from build123d import *

# Parameters (mm, degrees)
SKETCH1_W             = 60
SKETCH1_H             = 60
BOSS_EXTRUDE1_DEPTH   = 6
SKETCH2_W             = 55
SKETCH2_H             = 15.25
BOSS_EXTRUDE2_DEPTH   = 30
F_5_0MM_DOWEL_HOLE1_D = 5
FILLET1_R             = 5
F_5_0MM_DOWEL_HOLE2_D = 5


with BuildPart() as part:
    # Sketch1 → Boss-Extrude1 (new body)
    with BuildSketch(Plane.XY):
        Rectangle(SKETCH1_W, SKETCH1_H)
    extrude(amount=BOSS_EXTRUDE1_DEPTH)

    # Sketch2 → Boss-Extrude2 (add)
    with BuildSketch(Plane(origin=(0, 0, 0), x_dir=(-1, 0, 0), z_dir=(0, 0, -1))):
        Rectangle(SKETCH2_W, SKETCH2_H)
    extrude(amount=BOSS_EXTRUDE2_DEPTH)

    # Ø5.0mm Dowel Hole1 (through all)
    with Locations(Plane(origin=(0, 0, 0), x_dir=(-1, 0, 0), z_dir=(0, 0, -1))):
        with Locations((25, 25), (-25, 25), (25, -25), (-25, -25)):
            Hole(F_5_0MM_DOWEL_HOLE1_D / 2)

    # Fillet1
    fillet1_edges = [part.edges().sort_by_distance(p)[0] for p in [
        (30, -30, 3),
        (-30, -30, 3),
        (-30, 30, 3),
        (30, 30, 3),
    ]]
    fillet(fillet1_edges, radius=FILLET1_R)

    # Ø5.0mm Dowel Hole2 (through all)
    with Locations(Plane(origin=(0, 7.625, 0), x_dir=(1, 0, 0), z_dir=(0, 1, 0))):
        with Locations((20.5, 25), (20.5, 5), (-20.5, 5), (-20.5, 25)):
            Hole(F_5_0MM_DOWEL_HOLE2_D / 2)


solid = part.part
Verification items for the finished model (mm, model axes). A direction names the side the tool comes from. Give positions to 0.01 mm unless a question says otherwise; leave off trailing zeros. Order: outer loops, then holes, each group sorted by start corner. A loop starts at its lowest first (then second) coordinate and runs counter-clockwise, first axis right, second up. Notation, with made-up numbers: M 4,36 L 13,36 A25 ccw 13,50 Z; hole C 18,60.5 d10. An arc over 180 degrees is marked long. Use one line per item in the form item = value. Start each with the question number.
Q1. Section check A-A (z = -5). Enter the section's corners in (x, y) (3 decimals), then the cut area to 3 significant figures.
Q2. Go/stop test with flat-tipped pins: pin 1 Ø2 at (y, z) = (2, -7.5) entering from -X; pin 2 Ø8 at (x, z) = (-20.5, -5) entering from +Y (3 decimals); pin 3 Ø6 at (x, z) = (20.5, -5) entering from -Y (3 decimals); pin 4 Ø4 at (x, y) = (25, -25) entering from +Z. Record where each tip stops, or that it passes through.
Q3. Mould release check, pull along X, two halves, no side actions. Record for faces 3 (the cylindrical face through (24.67, -22.52, 3.04)), 4 (the flat face through (30, 0, 3)), 5 (the flat face through (0, -7.625, -15)): +X half, -X half, draft (parallel to the pull), parting line (faces both ways), or undercut.
Q4. Section check B-B (x = -20.5). Enter the section's corners in (y, z) (3 decimals).
Q5. Access from +Z, -Z, +X, -X, +Y, -Y to the whole of each face (thin tool, end or side, straight path). Record for faces 1 (the cylindrical face through (-29, 28, 3)), 2 (the flat face through (27.5, 0, -15)).
Q6. Section check C-C (y = -1.5). Enter the section's corners in (x, z).
Q7. Scan lines: line 1 along Y through (x, z) = (25, 3); line 2 along Z through (x, y) = (20.5, 3); line 3 along Y through (x, z) = (19, -13) (3 decimals). Record each from-to range of solid material in increasing order. Write a range as [from, to].
Q8. Section check D-D (y = 26.5). Enter the section's corners in (x, z), then the cut area to 3 significant figures.
Evaluation:
q1.outline = M -27.5,-7.625 L -23,-7.625 L -23,7.625 L -27.5,7.625 Z; M -18,-7.625 L 18,-7.625 L 18,7.625 L -18,7.625 Z; M 23,-7.625 L 27.5,-7.625 L 27.5,7.625 L 23,7.625 Z
q1.area = 686 mm2
q2.pin_1 = -27.5
q2.pin_2 = 7.625
q2.pin_3 = -7.625
q2.pin_4 = through
q3.face_3 = undercut
q3.face_4 = +X half
q3.face_5 = draft
q4.outline = M -30,0 L -7.625,0 L -7.625,-2.5 L 7.625,-2.5 L 7.625,0 L 30,0 L 30,6 L -30,6 Z; M -7.625,-30 L 7.625,-30 L 7.625,-27.5 L -7.625,-27.5 Z; M -7.625,-22.5 L 7.625,-22.5 L 7.625,-7.5 L -7.625,-7.5 Z
q5.face_1 = +Z, -Z, -X, +Y
q5.face_2 = -Z, +X, +Y, -Y
q6.outline = M -30,0 L -27.5,0 L -27.5,-30 L 27.5,-30 L 27.5,0 L 30,0 L 30,6 L -30,6 Z; hole C -20.5,-25 d5; hole C -20.5,-5 d5; hole C 20.5,-25 d5; hole C 20.5,-5 d5
q7.line_1 = [-30, -27.5], [-22.5, 22.5], [27.5, 30]
q7.line_2 = [-30, -27.5], [-22.5, -7.5], [-2.5, 6]
q7.line_3 = [-7.625, 7.625]
q8.outline = M -29.77,0 L -27,0 L -27,6 L -29.77,6 Z; M -23,0 L 23,0 L 23,6 L -23,6 Z; M 27,0 L 29.77,0 L 29.77,6 L 27,6 Z
q8.area = 309 mm2
